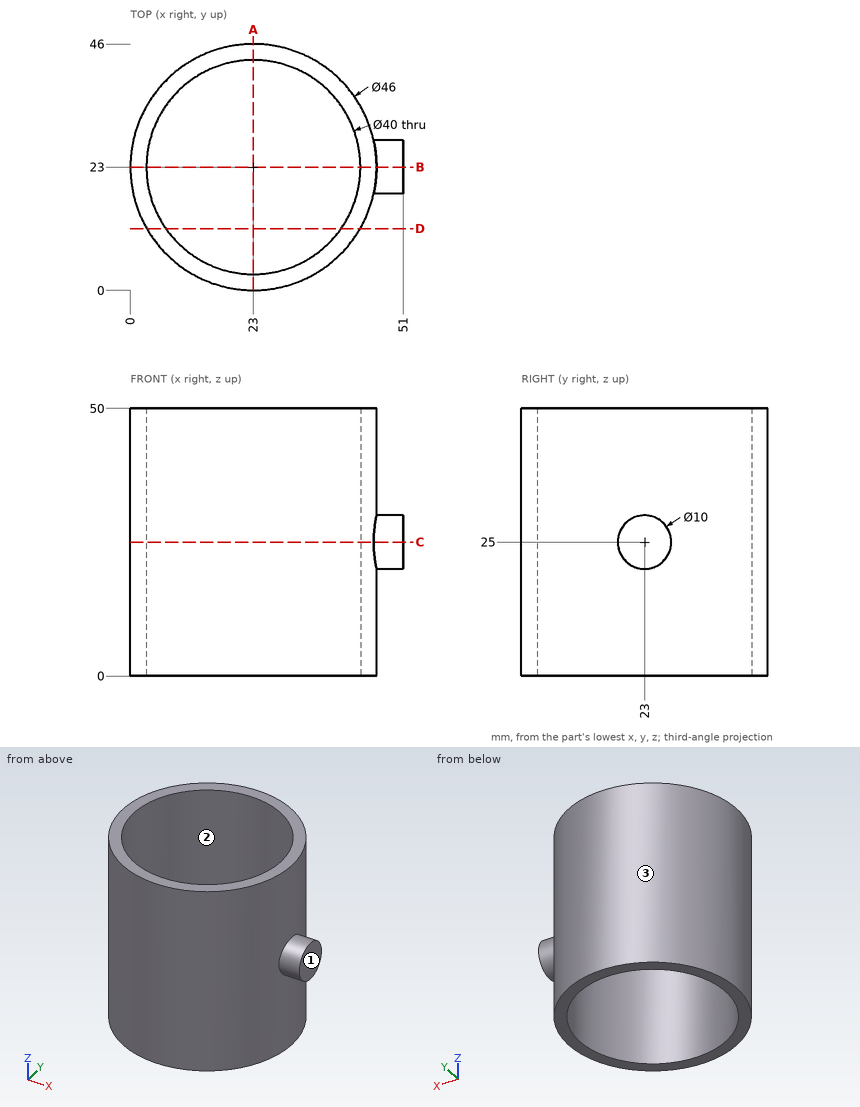
For this review, use the dimensioned drawing (mm, ordinates from the lowest corner) and the shaded views. Round coordinates to 2 decimals unless told otherwise and drop trailing zeros. Write each loop counter-clockwise with the first axis right and the second up, starting at its lowest first coordinate (ties: lowest second). Pieces come first, ordered by that corner, then holes. Notation, with made-up numbers: (36, 12.5) -> (54, 12.5) arc R28 cw to (54, 38.5) -> close; hole circle Ø2 at (-14, 41). An arc over 180 degrees is marked (long way). Use CSV: the item, a comma, the result in double quotes.
Q1. Consider section C-C (z = 25). Give the boundary of the cut face in (x, y).
Checks:
outline,"(45.45, 18) -> (51, 18) -> (51, 28) -> (45.45, 28) arc R23 ccw (long way) to start; hole circle Ø40 at (23, 23)"
Q2. Mouldability with a two-part tool opening along X and no side actions: class the marked faces 1, 2 and 3 as released by +X, released by -X, zero draft, split by the parting line, or undercut.
Checks:
face 1,"released by +X"
face 2,"undercut"
face 3,"split by the parting line"
Q3. To check wall thickness, follow probe 1 along Y at (x, z) = (23, 22); probe 2 along Y at (x, z) = (18.5, 43.5); probe 3 along X at (y, z) = (11.5, 37.5). State the ranges of each line that lie inside material, in increasing order. Write a range as [from, to].
Checks:
probe 1,"[0, 3], [43, 46]"
probe 2,"[0.44, 3.51], [42.49, 45.56]"
probe 3,"[3.08, 6.64], [39.36, 42.92]"
Q4. Consider section B-B (y = 23). Give the boundary of the cut face in (x, z), then the cut area to 3 significant figures.
Checks:
outline,"(0, 0) -> (3, 0) -> (3, 50) -> (0, 50) -> close; (43, 0) -> (46, 0) -> (46, 20) -> (51, 20) -> (51, 30) -> (46, 30) -> (46, 50) -> (43, 50) -> close"
area,"350 mm²"
Q5. Consider section A-A (x = 23). Give the boundary of the cut face in (y, z).
Checks:
outline,"(0, 0) -> (3, 0) -> (3, 50) -> (0, 50) -> close; (43, 0) -> (46, 0) -> (46, 50) -> (43, 50) -> close"
Q6. For pin 1 Ø3 at (y, z) = (12, 37.5) entering from +X; pin 2 Ø1 at (y, z) = (30, 16) entering from -X; pin 3 Ø12 at (y, z) = (19.5, 13.5) entering from -X; pin 4 Ø12 at (x, z) = (19.5, 40) entering from -Y, all flat-tipped, find the tip position at first contact; note any pin that passes through.
Checks:
pin 1,"x = 43.95"
pin 2,"x = 0.94"
pin 3,"x = 0"
pin 4,"y = 0"
Q7. Consider section D-D (y = 11.5). Give the boundary of the cut face in (x, z).
Checks:
outline,"(3.08, 0) -> (6.64, 0) -> (6.64, 50) -> (3.08, 50) -> close; (39.36, 0) -> (42.92, 0) -> (42.92, 50) -> (39.36, 50) -> close"
